Model file for the job. Use its own axes, mm. A direction names the side the tool comes from. Coordinates: 2 decimals unless noted, no trailing zeros. Write each loop counter-clockwise with the first axis right and the second up, starting at its lowest first coordinate (ties: lowest second). Pieces come first, ordered by that corner, then holes. Notation, with made-up numbers: M 16,-5 L 38,-5 A19 cw 38,18 Z; hole C 52,38 d2. An arc over 180 degrees is marked long. One line per question, with ' | ' between items. Start each with the question number.
(1) Tool access for faces 4 (the face through (4.676, 2.21, 1.263)), 5 (the face through (4, 0, 52)), 6 (the face through (2, 1, 95.5)): list every direction of +Z, -Z, +X, -X, +Y, -Y with a clear straight run to the whole face (end or side of a thin tool).
(2) Flat gauge pin, fed straight in: pin 1 Ø0.6 at (x, z) = (3.5, 98) entering from +Y. Where does the tip first touch, or does it go through?
(3) Two-plate mould, pull along X, no slides. Class faces 1 (the face through (0, 1, 54)), 2 (the face through (4, 2.95, 52)), 3 (the face through (4, 2, 97)): +X half, -X half, draft (parallel to the pull), parting line (faces both ways), or undercut.
(4) Wall check: probe 1 along X at (y, z) = (0.95, 98); probe 2 along X at (y, z) = (2.25, 104); probe 3 along Z at (x, y) = (4.5, 2.7). Give the ranges that are in metal, low to high.
(5) Cut at A-A (y = 2.45). Write the cut outline in (x, z), plus the area to 3 significant figures.
from build123d import *

# Parameters (mm, degrees)
SKETCH_1_W          = 8
SKETCH_1_H          = 106
EXTRUDE_1_DEPTH     = 2.95
SKETCH_2_R          = 0.7
CUT_EXTRUDE_1_DEPTH = 107.342383366
SKETCH_2_3_R        = 1
CUT_EXTRUDE_2_DEPTH = 1.5
SKETCH_3_W          = 1.6
SKETCH_3_H          = 1.2
CUT_EXTRUDE_3_DEPTH = 107.342383366


with BuildPart() as part:
    # Sketch 1 → Extrude 1 (new body)
    with BuildSketch(Plane(origin=(0, 0, 0), x_dir=(1, 0, 0), z_dir=(0, 1, 0))):
        with Locations((4, -53)):
            Rectangle(SKETCH_1_W, SKETCH_1_H)
    extrude(amount=EXTRUDE_1_DEPTH)

    # Sketch 2 → Cut-Extrude 1 (cut, through all)
    with BuildSketch(Plane(origin=(0, 2.95, 0), x_dir=(1, 0, 0), z_dir=(0, 1, 0))):
        with Locations(Location((4, -8, 0), (0, 0, 270))):
            Circle(SKETCH_2_R)
        with Locations(Location((4, -2, 0), (0, 0, 270))):
            Circle(SKETCH_2_R)
        with Locations(Location((4, -104, 0), (0, 0, 270))):
            Circle(SKETCH_2_R)
        with Locations(Location((4, -98, 0), (0, 0, 270))):
            Circle(SKETCH_2_R)
        with Locations(Location((4, -28, 0), (0, 0, 270))):
            Circle(SKETCH_2_R)
    extrude(amount=-CUT_EXTRUDE_1_DEPTH, mode=Mode.SUBTRACT)

    # Sketch 2_3 → Cut-Extrude 2 (cut)
    with BuildSketch(Plane(origin=(0, 2.95, 0), x_dir=(1, 0, 0), z_dir=(0, 1, 0))):
        with Locations(Location((4, -8, 0), (0, 0, 270))):
            Circle(SKETCH_2_3_R)
        with Locations(Location((4, -2, 0), (0, 0, 270))):
            Circle(SKETCH_2_3_R)
        with Locations(Location((4, -104, 0), (0, 0, 270))):
            Circle(SKETCH_2_3_R)
        with Locations(Location((4, -98, 0), (0, 0, 270))):
            Circle(SKETCH_2_3_R)
        with Locations(Location((4, -28, 0), (0, 0, 270))):
            Circle(SKETCH_2_3_R)
    extrude(amount=-CUT_EXTRUDE_2_DEPTH, mode=Mode.SUBTRACT)

    # Sketch 3 → Cut-Extrude 3 (cut, through all)
    with BuildSketch(Plane(origin=(0, 2.95, 0), x_dir=(1, 0, 0), z_dir=(0, 1, 0))):
        with Locations((1.8, -94.9)):
            Rectangle(SKETCH_3_W, SKETCH_3_H)
        with Locations((6.2, -94.9)):
            Rectangle(SKETCH_3_W, SKETCH_3_H)
    extrude(amount=-CUT_EXTRUDE_3_DEPTH, mode=Mode.SUBTRACT)


solid = part.part
Filled in:
1) face 4: +Y | face 5: +Z, -Z, +X, -X, -Y | face 6: +Y, -Y
2) pin 1: y = 1.45
3) face 1: -X half | face 2: draft | face 3: undercut
4) probe 1: 0 to 3.3, 4.7 to 8 | probe 2: 0 to 3, 5 to 8 | probe 3: 0 to 1.13, 2.87 to 7.13, 8.87 to 27.13, 28.87 to 97.13, 98.87 to 103.13, 104.87 to 106
5) outline: M 0,0 L 8,0 L 8,106 L 0,106 Z; hole M 1,94.3 L 2.6,94.3 L 2.6,95.5 L 1,95.5 Z; hole C 4,2 d2; hole C 4,8 d2; hole C 4,28 d2; hole C 4,98 d2; hole C 4,104 d2; hole M 5.4,94.3 L 7,94.3 L 7,95.5 L 5.4,95.5 Z | area: 828 mm²
